Could you check a few things on this model? Use its own coordinates, in mm. A direction names the side the tool comes from. Round coordinates to 2 decimals unless told otherwise and drop trailing zeros. Write each loop counter-clockwise with the first axis right and the second up, starting at its lowest first coordinate (ties: lowest second). Pieces come first, ordered by that corner, then holes. Notation, with made-up numbers: (41, 47.5) -> (54, 47.5) arc R28 ccw to (54, 83.5) -> close; hole circle Ø10 at (-7.5, 59.25). An arc over 180 degrees is marked (long way). Answer in a Markdown table with one row per item. Add a question column.
```python
from build123d import *
from OCP.BRepFilletAPI import BRepFilletAPI_MakeChamfer

# Parameters (mm, degrees)
SKETCH1_R                 = 6.1
BOSS_EXTRUDE1_DEPTH       = 1.3
SKETCH2_R                 = 2.85
BOSS_EXTRUDE2_DEPTH       = 0.3
SKETCH5_R                 = 3.45
BOSS_EXTRUDE3_DEPTH       = 0.2
F_2_0MM_DOWEL_HOLE1_D     = 2
F_2_0MM_DOWEL_HOLE1_DEPTH = 52.32
F_2_0MM_DOWEL_HOLE1_TIP   = 0.600860619
SKETCH6_R                 = 2.6
SKETCH6_R_2               = 2.1
BOSS_EXTRUDE4_DEPTH       = 0.8
CUT_EXTRUDE1_START        = -1.6
SKETCH8_R                 = 2.1
CUT_EXTRUDE1_DEPTH        = 1.6
BOSS_EXTRUDE5_DEPTH       = 1.9
BOSS_EXTRUDE5_DEPTH_BACK  = 0.6
SKETCH9_W                 = 6.5
SKETCH9_H                 = 3
CHAMFER1_SIZE             = 1
CHAMFER1_SIZE2            = 1.732050808
CUT_EXTRUDE2_DEPTH        = 12.405919516
CUT_EXTRUDE2_DEPTH_BACK   = 12.405919516
BOSS_EXTRUDE6_DEPTH       = 2.2
BOSS_EXTRUDE6_DEPTH_BACK  = 2
BOSS_EXTRUDE6_START       = 0.65
CUT_EXTRUDE3_DEPTH        = 10
FILLET1_R                 = 0.25


with BuildPart() as part:
    # Sketch1 → Boss-Extrude1 (new body)
    with BuildSketch(Plane(origin=(0, 0, 0), x_dir=(1, 0, 0), z_dir=(0, 1, 0))):
        with Locations(Location((0, 0, 0), (0, 0, 270))):
            Circle(SKETCH1_R)
    extrude(amount=BOSS_EXTRUDE1_DEPTH)

    # Sketch2 → Boss-Extrude2 (add)
    with BuildSketch(Plane(origin=(0, 1.3, 0), x_dir=(1, 0, 0), z_dir=(0, 1, 0))):
        with Locations(Location((0, 0, 0), (0, 0, 270))):
            Circle(SKETCH2_R)
    extrude(amount=BOSS_EXTRUDE2_DEPTH)

    # Sketch5 → Boss-Extrude3 (add)
    with BuildSketch(Plane.XZ):
        with Locations(Location((0, 0, 0), (0, 0, 270))):
            Circle(SKETCH5_R)
    extrude(amount=BOSS_EXTRUDE3_DEPTH)

    # Ø2.0mm Dowel Hole1
    with Locations(Plane(origin=(0, 1.6, 0), x_dir=(1, 0, 0), z_dir=(0, 1, 0))):
        with Locations((0, 0)):
            Hole(F_2_0MM_DOWEL_HOLE1_D / 2, depth=F_2_0MM_DOWEL_HOLE1_DEPTH)
            with Locations((0, 0, -(F_2_0MM_DOWEL_HOLE1_DEPTH + F_2_0MM_DOWEL_HOLE1_TIP / 2))):  # 118° drill point
                Cone(0, F_2_0MM_DOWEL_HOLE1_D / 2, F_2_0MM_DOWEL_HOLE1_TIP, mode=Mode.SUBTRACT)

    # Sketch6 → Boss-Extrude4 (add)
    with BuildSketch(Plane.XZ.offset(0.2)):
        with Locations(Location((0, 0, 0), (0, 0, 270))):
            Circle(SKETCH6_R)
        with Locations(Location((0, 0, 0), (0, 0, 270))):
            Circle(SKETCH6_R_2, mode=Mode.SUBTRACT)
    extrude(amount=BOSS_EXTRUDE4_DEPTH)

    # Sketch8 → Cut-Extrude1 (cut)
    with BuildSketch(Plane.XZ.offset(1).offset(CUT_EXTRUDE1_START)):
        with Locations(Location((0, 0, 0), (0, 0, 270))):
            Circle(SKETCH8_R)
    extrude(amount=CUT_EXTRUDE1_DEPTH, mode=Mode.SUBTRACT)

    # Sketch9 → Boss-Extrude5 (add, two sides: drawn at the far end of the back side and taken through both)
    with BuildSketch(Plane(origin=(0, 0, 0), x_dir=(1, 0, 0), z_dir=(0, 1, 0)).offset(-BOSS_EXTRUDE5_DEPTH_BACK)):
        with Locations((0, 4.75)):
            Rectangle(SKETCH9_W, SKETCH9_H)
    extrude(amount=BOSS_EXTRUDE5_DEPTH + BOSS_EXTRUDE5_DEPTH_BACK)

    # Chamfer1: one chamfer whose edges measure the first distance from different faces: ONE call of the kernel's chamfer builder (chamfer() names one face for all edges)
    chamfer1_edges_1 = [part.edges().sort_by_distance(p)[0] for p in [
        (3.25, -0.3, -3.25),
        (3.25, 1.6, -3.25),
    ]]
    chamfer1_side_1 = [part.faces().sort_by_distance(p)[0] for p in [
        (3.25, 1.6, -3.289051248),
    ]]
    chamfer1_edges_2 = [part.edges().sort_by_distance(p)[0] for p in [
        (-3.25, 1.6, -3.25),
        (-3.25, -0.3, -3.25),
    ]]
    chamfer1_side_2 = [part.faces().sort_by_distance(p)[0] for p in [
        (-3.25, 0.65, -6.210948752),
    ]]
    chamfer1 = BRepFilletAPI_MakeChamfer(part.part.solid().wrapped)
    for e in chamfer1_edges_1:
        chamfer1.Add(CHAMFER1_SIZE, CHAMFER1_SIZE2, e.wrapped, chamfer1_side_1[0].wrapped)  # the first distance lies on this face
    for e in chamfer1_edges_2:
        chamfer1.Add(CHAMFER1_SIZE, CHAMFER1_SIZE2, e.wrapped, chamfer1_side_2[0].wrapped)  # the first distance lies on this face
    add(Compound.cast(chamfer1.Shape()), mode=Mode.REPLACE)

    # Sketch10 → Cut-Extrude2 (cut, two sides: drawn at the far end of the back side and taken through both)
    with BuildSketch(Plane(origin=(3.25, 0, 0), x_dir=(0, 0, -1), z_dir=(1, 0, 0)).offset(-CUT_EXTRUDE2_DEPTH_BACK)):
        Polygon((3.25, 1.500247446), (6.25, 1.9), (3.25, 1.9), align=None)
        Polygon((3.25, -0.6), (6.25, -0.6), (3.25, -0.2), align=None)
    extrude(amount=CUT_EXTRUDE2_DEPTH + CUT_EXTRUDE2_DEPTH_BACK, mode=Mode.SUBTRACT)

    # Sketch11 → Boss-Extrude6 (add, two sides: drawn at the far end of the back side and taken through both)
    with BuildSketch(Plane(origin=(0, 0, 0), x_dir=(1, 0, 0), z_dir=(0, 1, 0)).offset(BOSS_EXTRUDE6_START - BOSS_EXTRUDE6_DEPTH_BACK)):
        with BuildLine():
            Line((-2.15, 7.185227902), (-2.15, 4.185227902))
            Line((-2.15, 4.185227902), (-0.85, 4.185227902))
            Line((-0.85, 4.185227902), (-0.85, 5.425500648))
            Line((-0.85, 5.425500648), (0.85, 5.425500648))
            Line((0.85, 5.425500648), (0.85, 4.185227902))
            Line((0.85, 4.185227902), (2.15, 4.185227902))
            Line((2.15, 4.185227902), (2.15, 7.185227902))
            ThreePointArc((2.15, 7.185227902), (0, 7.5), (-2.15, 7.185227902))
        make_face()
    extrude(amount=BOSS_EXTRUDE6_DEPTH + BOSS_EXTRUDE6_DEPTH_BACK)

    # Sketch12 → Cut-Extrude3 (cut)
    with BuildSketch(Plane.ZY.offset(2.15)):
        with BuildLine():
            Line((-7.185227902, 2.85), (-4.185227902, 2.85))
            Line((-4.185227902, 2.85), (-4.185227902, 2.05486736))
            ThreePointArc((-4.185227902, 2.05486736), (-5.650660459, 2.582855102), (-7.185227902, 2.85))
        make_face()
        with BuildLine():
            Line((-4.185227902, -0.754697054), (-4.185227902, -1.35))
            Line((-4.185227902, -1.35), (-7.185227902, -1.35))
            ThreePointArc((-7.185227902, -1.35), (-5.659726016, -1.180864031), (-4.185227902, -0.754697054))
        make_face()
    extrude(amount=-CUT_EXTRUDE3_DEPTH, mode=Mode.SUBTRACT)

    # Fillet1
    fillet1_edges = [part.edges().sort_by_distance(p)[0] for p in [
        (-3.25, 0.65, -6.25),
        (3.25, 0.65, -6.25),
    ]]
    fillet(fillet1_edges, radius=FILLET1_R)


solid = part.part
```
(1) I need wall thicknesses on L1, parallel to Z at x = 0, y = 1.15; L2, parallel to X at y = 1.85, z = -4.25; L3, parallel to Y at x = -4.5, z = -1.75. Which ranges of each line are inside material? Lowest first, please.
(2) For P1, Ø0.5, axis at y = 1, z = -5.5, coming from the -X side; P2, Ø5.5, axis at x = 0, z = 0, coming from the +Y side; P3, Ø1.5, axis at y = -0.5, z = 2, coming from the +X side, each with a flat end and sliding along its axis, tell me the tip position at first contact or that it passes through.
(3) Suppose I cut it at C-C, the plane y = 0.15. Please give me the cut outline in (x, z), then the cut area to 3 significant figures.
(4) If we mould it in two halves opening along X, with no side actions, what happens to faces 1 (the face through (0.631, -0.189, -2.003)), 2 (the face through (3.25, 0.6, -5.5)), 3 (the face through (-3.25, 0.6, -5.5)), 4 (the face through (0.78, -0.59, -2.48))? For each: pulls with the +X half, pulls with the -X half, needs draft (parallel to the pull), parting line crosses it, or undercut.
(5) Suppose I cut it at A-A, the plane z = 0. Please give me the cut outline in (x, y).
(6) Suppose I cut it at D-D, the plane z = -4.5. Please give me the cut outline in (x, y).
(7) On a 3-axis mill with a long thin cutter (end or side, diameter ignored), from which of +Z, -Z, +X, -X, +Y, -Y can I reach the whole of each face in a straight line? I mean faces 5 (the face through (0.85, 2, -5)), 6 (the face through (-3, -0.2, 1)), 7 (the face through (-2.6, 0.6, -6.25)), 8 (the face through (-0.22, 0.641, 6.096)), 9 (the face through (-2.78, 1.45, -0.62)). Say none if no direction works.
Response:
| question | item | result |
|---|---|---|
| 1 | L1 | -7.5 to -1, 1 to 6.1 |
| 1 | L2 | -2.15 to -0.85, 0.85 to 2.15 |
| 1 | L3 | 0 to 1.3 |
| 2 | P1 | x = -3.25 |
| 2 | P2 | y = 1.6 |
| 2 | P3 | x = 5.93 |
| 3 | outline | (-3.25, -6) arc R0.25 ccw to (-3, -6.25) -> (-2.15, -6.25) -> (-2.15, -7.19) arc R7.5 ccw to (2.15, -7.19) -> (2.15, -6.25) -> (3, -6.25) arc R0.25 ccw to (3.25, -6) -> (3.25, -5.16) arc R6.1 ccw (long way) to (-3.25, -5.16) -> close; hole circle Ø4.2 at (0, 0) |
| 3 | area | 111 mm² |
| 4 | face 1 | undercut |
| 4 | face 2 | pulls with the +X half |
| 4 | face 3 | pulls with the -X half |
| 4 | face 4 | parting line crosses it |
| 5 | outline | (-6.1, 0) -> (-3.45, 0) -> (-3.45, -0.2) -> (-2.6, -0.2) -> (-2.6, -1) -> (-2.1, -1) -> (-2.1, 0.6) -> (-1, 0.6) -> (-1, 1.6) -> (-2.85, 1.6) -> (-2.85, 1.3) -> (-6.1, 1.3) -> close; (1, 0.6) -> (2.1, 0.6) -> (2.1, -1) -> (2.6, -1) -> (2.6, -0.2) -> (3.45, -0.2) -> (3.45, 0) -> (6.1, 0) -> (6.1, 1.3) -> (2.85, 1.3) -> (2.85, 1.6) -> (1, 1.6) -> close |
| 6 | outline | (-4.12, 0) -> (-3.25, 0) -> (-3.25, -0.37) -> (-2.15, -0.37) -> (-2.15, -0.87) -> (-0.85, -0.87) -> (-0.85, -0.37) -> (0.85, -0.37) -> (0.85, -0.87) -> (2.15, -0.87) -> (2.15, -0.37) -> (3.25, -0.37) -> (3.25, 0) -> (4.12, 0) -> (4.12, 1.3) -> (3.25, 1.3) -> (3.25, 1.67) -> (2.15, 1.67) -> (2.15, 2.19) -> (0.85, 2.19) -> (0.85, 1.67) -> (-0.85, 1.67) -> (-0.85, 2.19) -> (-2.15, 2.19) -> (-2.15, 1.67) -> (-3.25, 1.67) -> (-3.25, 1.3) -> (-4.12, 1.3) -> close |
| 7 | face 5 | +Z, +Y |
| 7 | face 6 | -Y |
| 7 | face 7 | -Z, -X, +Y, -Y |
| 7 | face 8 | +Y, -Y |
| 7 | face 9 | +Y |
